from build123d import *

# Parameters (mm, degrees)
F1_DEPTH = 31.6
F2_START = 27.6
F2_DEPTH = 4
F0_R     = 3.05
F3_DEPTH = 2
F4_W     = 2.5
F4_H     = 29.6
F5_DEPTH = 2
F7_DEPTH = 3
F8_R     = 0.5
F9_DEPTH = 25


with BuildPart() as f1:
    # F0 (on Top) → F1 (new body)
    with BuildSketch(Plane.XY):
        Polygon((31.25, -9), (31.25, 0), (29.25, 0), (29.25, -7), (-29.25, -7), (-29.25, 0), (-31.25, 0), (-31.25, -9), align=None)
        Polygon((31.25, 0), (31.25, 9), (-31.25, 9), (-31.25, 0), (-29.25, 0), (-29.25, 7), (29.25, 7), (29.25, 0), align=None)
    extrude(amount=F1_DEPTH)

    # F0 (on Top) → F2 (join)
    with BuildSketch(Plane.XY.offset(F2_START)):
        with BuildLine():
            Line((29, 0), (29.25, 0))
            Line((29.25, 0), (29.25, 7))
            Line((29.25, 7), (-29.25, 7))
            Line((-29.25, 7), (-29.25, 0))
            Line((-29.25, 0), (-29, 0))
            ThreePointArc((-29, 0), (-24.5, 4.5), (-20, 0))
            Line((-20, 0), (-16.1, 0))
            ThreePointArc((-16.1, 0), (-13.5, 2.6), (-10.9, 0))
            Line((-10.9, 0), (-7.1, 0))
            ThreePointArc((-7.1, 0), (-4.5, 2.6), (-1.9, 0))
            Line((-1.9, 0), (0, 0))
            Line((0, 0), (1.9, 0))
            ThreePointArc((1.9, 0), (4.5, 2.6), (7.1, 0))
            Line((7.1, 0), (10.9, 0))
            ThreePointArc((10.9, 0), (13.5, 2.6), (16.1, 0))
            Line((16.1, 0), (20, 0))
            ThreePointArc((20, 0), (24.5, 4.5), (29, 0))
        make_face()
        with BuildLine():
            Line((29.25, -7), (29.25, 0))
            Line((29.25, 0), (29, 0))
            ThreePointArc((29, 0), (24.5, -4.5), (20, 0))
            Line((20, 0), (16.1, 0))
            ThreePointArc((16.1, 0), (13.5, -2.6), (10.9, 0))
            Line((10.9, 0), (7.1, 0))
            ThreePointArc((7.1, 0), (4.5, -2.6), (1.9, 0))
            Line((1.9, 0), (0, 0))
            Line((0, 0), (-1.9, 0))
            ThreePointArc((-1.9, 0), (-4.5, -2.6), (-7.1, 0))
            Line((-7.1, 0), (-10.9, 0))
            ThreePointArc((-10.9, 0), (-13.5, -2.6), (-16.1, 0))
            Line((-16.1, 0), (-20, 0))
            ThreePointArc((-20, 0), (-24.5, -4.5), (-29, 0))
            Line((-29, 0), (-29.25, 0))
            Line((-29.25, 0), (-29.25, -7))
            Line((-29.25, -7), (29.25, -7))
        make_face()
    extrude(amount=F2_DEPTH)

    # F0 (on Top) → F3 (join)
    with BuildSketch(Plane.XY):
        Polygon((-41.25, 19), (-41.25, 14), (-41.25, -19), (41.25, -19), (41.25, 19), align=None)
        with Locations((-27.5, 14)):
            Circle(F0_R, mode=Mode.SUBTRACT)
        Polygon((-31.25, 9), (31.25, 9), (31.25, 0), (31.25, -9), (-31.25, -9), (-31.25, 0), align=None, mode=Mode.SUBTRACT)
        with Locations((27.5, 14)):
            Circle(F0_R, mode=Mode.SUBTRACT)
    extrude(amount=F3_DEPTH)

    # F4 (on face) → F5 (cut)
    with BuildSketch(Plane.XZ.offset(9)):
        with Locations((-1.25, 16.8)):
            Rectangle(F4_W, F4_H)
        with Locations((1.25, 16.8)):
            Rectangle(F4_W, F4_H)
        with Locations((-19.25, 16.8)):
            Rectangle(F4_W, F4_H)
        with Locations((-16.75, 16.8)):
            Rectangle(F4_W, F4_H)
        with Locations((-10.25, 16.8)):
            Rectangle(F4_W, F4_H)
        with Locations((-7.75, 16.8)):
            Rectangle(F4_W, F4_H)
        with Locations((10.25, 16.8)):
            Rectangle(F4_W, F4_H)
        with Locations((7.75, 16.8)):
            Rectangle(F4_W, F4_H)
        with Locations((16.75, 16.8)):
            Rectangle(F4_W, F4_H)
        with Locations((19.25, 16.8)):
            Rectangle(F4_W, F4_H)
    extrude(amount=-F5_DEPTH, mode=Mode.SUBTRACT)

    # F6 (on face) → F7 (join)
    with BuildSketch(Plane.XY.offset(31.6)):
        Polygon((-27, -6), (-27, -9), (-25, -9), (-23, -9), (-23, -6), (-25, -6), align=None)
        Polygon((23, -6), (23, -9), (25, -9), (27, -9), (27, -6), (25, -6), align=None)
        Polygon((-23, 6), (-23, 9), (-25, 9), (-27, 9), (-27, 6), (-25, 6), align=None)
        Polygon((25, 6), (27, 6), (27, 9), (25, 9), (23, 9), (23, 6), align=None)
    extrude(amount=F7_DEPTH)

    # F8 (on face) → F9 (cut)
    with BuildSketch(Plane.XZ.offset(9)):
        with BuildLine():
            ThreePointArc((-25, 33.6), (-25.3535533906, 32.7464466094), (-24.5, 33.1))
            ThreePointArc((-24.5, 33.1), (-24.6464466094, 33.4535533906), (-25, 33.6))
        make_face()
        with Locations((25, 33.1)):
            Circle(F8_R)
    extrude(amount=-F9_DEPTH, mode=Mode.SUBTRACT)


solid = f1.part
Part model, mm, in its own coordinate system. A direction names the side the tool comes from. Give positions to 0.01 mm unless a question says otherwise; leave off trailing zeros. Order: outer loops, then holes, each group sorted by start corner. A loop starts at its lowest first (then second) coordinate and runs counter-clockwise, first axis right, second up. Notation, with made-up numbers: (53, 67) - (80, 67) arc R25 cw to (80, 86) - close; hole circle Ø7 at (-33.5, 69). An arc over 180 degrees is marked (long way). Use a Markdown table: item, result.
1) Saw through at D-D on y = 15. List the corners of the cut face in (x, z).
Checked values:
| item | result |
|---|---|
| outline | (-41.25, 0) - (-30.38, 0) - (-30.38, 2) - (-41.25, 2) - close; (-24.62, 0) - (24.62, 0) - (24.62, 2) - (-24.62, 2) - close; (30.38, 0) - (41.25, 0) - (41.25, 2) - (30.38, 2) - close |
2) Saw through at C-C on z = 30.5. Count the separate pieces of the cut face and the enclosed holes in it, plus the area to 3 significant figures.
Checked values:
| item | result |
|---|---|
| separate pieces | 1 |
| enclosed holes | 6 |
| area | 863 mm² |
3) 3-axis set-ups, long thin cutter, end or side, ignore diameter. For faces 4 (the flat face through (-31.25, 0, 17)), 5 (the flat face through (-23, 7, 33)), 6 (the flat face through (4, -9, 17)), 7 (the flat face through (-6.5, -8, 17)), 8 (the flat face through (29.25, 0, 14)): which of +Z, -Z, +X, -X, +Y, -Y reach the whole face in a straight line?
Checked values:
| item | result |
|---|---|
| face 4 | +Z, -X, +Y, -Y |
| face 5 | +Z, +Y, -Y |
| face 6 | +Z, +X, -X, -Y |
| face 7 | +Z, -Y |
| face 8 | -Z |
4) Saw through at A-A on z = 6.5. List the corners of the cut face in (x, y).
Checked values:
| item | result |
|---|---|
| outline | (-31.25, -9) - (-20.5, -9) - (-20.5, -7) - (-29.25, -7) - (-29.25, 7) - (29.25, 7) - (29.25, -7) - (20.5, -7) - (20.5, -9) - (31.25, -9) - (31.25, 9) - (-31.25, 9) - close; (-15.5, -9) - (-11.5, -9) - (-11.5, -7) - (-15.5, -7) - close; (-6.5, -9) - (-2.5, -9) - (-2.5, -7) - (-6.5, -7) - close; (2.5, -9) - (6.5, -9) - (6.5, -7) - (2.5, -7) - close; (11.5, -9) - (15.5, -9) - (15.5, -7) - (11.5, -7) - close |
5) Two-plate mould, pull along Y, no slides. Class faces 1 (the cylindrical face through (-11.02, -0.78, 29.57)), 2 (the flat face through (0, 9, 18)), 3 (the flat face through (-26, -9, 18)): +Y half, -Y half, draft (parallel to the pull), parting line (faces both ways), or undercut.
Checked values:
| item | result |
|---|---|
| face 1 | undercut |
| face 2 | +Y half |
| face 3 | -Y half |
6) Saw through at B-B on x = -13.5. List the corners of the cut face in (y, z), plus the area to 3 significant figures.
Checked values:
| item | result |
|---|---|
| outline | (-19, 0) - (-7, 0) - (-7, 27.6) - (-2.6, 27.6) - (-2.6, 31.6) - (-9, 31.6) - (-9, 2) - (-19, 2) - close; (2.6, 27.6) - (7, 27.6) - (7, 0) - (19, 0) - (19, 2) - (9, 2) - (9, 31.6) - (2.6, 31.6) - close |
| area | 202 mm² |
7) Flat gauge pins, fed straight in: P1, Ø7, axis at x = 27.5, y = 14, coming from the -Z side; P2, Ø4, axis at x = -13.5, y = 0, coming from the +Z side; P3, Ø3, axis at x = 22, y = 4.5, coming from the -Z side; P4, Ø10, axis at x = -22, z = 18, coming from the +Y side. Where does each tip first touch, or does it go through?
Checked values:
| item | result |
|---|---|
| P1 | z = 0 |
| P2 | through |
| P3 | z = 27.6 |
| P4 | y = 9 |
8) Probe L1, parallel to Y at x = 24.5, z = 28.9; L2, parallel to X at y = 2.5, z = 25.5; L3, parallel to Z at x = 17.5, y = -15.5. List the from-to ranges inside material, lowest first. Write a range as from..to.
Checked values:
| item | result |
|---|---|
| L1 | -9..-4.5, 4.5..9 |
| L2 | -31.25..-29.25, 29.25..31.25 |
| L3 | 0..2 |
